Could you check a few things on this model? Use its own coordinates, in mm. Face numbers are marked on the shaded views. A direction names the side the tool comes from. Round coordinates to 2 decimals unless told otherwise and drop trailing zeros. Write each loop counter-clockwise with the first axis right and the second up, starting at its lowest first coordinate (ties: lowest second). Pieces come first, ordered by that corner, then holes. Notation, with made-up numbers: (58.25, 38.5) -> (83.25, 38.5) arc R14 ccw to (83.25, 63.5) -> close; hole circle Ø10 at (-11.75, 8). An arc over 180 degrees is marked (long way). Answer in a Markdown table with one row per item.
from build123d import *

# Parameters (mm, degrees)
SKETCH1_W           = 120
SKETCH1_H           = 37.194444444
BOSS_EXTRUDE4_DEPTH = 20
CUT_EXTRUDE15_DEPTH = 23
SKETCH10_W          = 11.898671916
SKETCH10_H          = 26.611218947
SKETCH10_W_2        = 10.049553983
SKETCH10_H_2        = 23.877740264
BOSS_EXTRUDE5_DEPTH = 30
SKETCH11_W          = 5.024776991
SKETCH11_H          = 23.877740264
BOSS_EXTRUDE6_DEPTH = 30
SKETCH12_W          = 4.765877192
SKETCH12_H          = 4.013370267
SKETCH12_H_2        = 4.515041551
CUT_EXTRUDE16_DEPTH = 16.868939526
FILLET2_R           = 5
SKETCH16_W          = 46.35727902
SKETCH16_H          = 19.765742142
CUT_EXTRUDE17_DEPTH = 5
FILLET3_R           = 5


with BuildPart() as part:
    # Sketch1 → Boss-Extrude4 (new body)
    with BuildSketch(Plane.XY):
        Polygon((36.833333333, 25.458333333), (36.833333333, 18.597222222), (60, 18.597222222), (60, -18.597222222), (68.25, -18.597222222), (72.583333333, 25.458333333), align=None)
        Rectangle(SKETCH1_W, SKETCH1_H)
    extrude(amount=BOSS_EXTRUDE4_DEPTH)

    # Sketch6 → Cut-Extrude15 (cut)
    with BuildSketch(Plane.XY.offset(20)):
        Polygon((51.910176302, 18.597222222), (36.833333333, 18.597222222), (36.833333333, 25.458333333), (72.583333333, 25.458333333), (68.25, -18.597222222), (55.010463364, -18.597222222), (60.177305366, 10.330093158), align=None)
    extrude(amount=-CUT_EXTRUDE15_DEPTH, mode=Mode.SUBTRACT)

    # Sketch10 → Boss-Extrude5 (add)
    with BuildSketch(Plane.ZY.offset(60)):
        with Locations((10.080396432, 0.080396432)):
            Rectangle(SKETCH10_W, SKETCH10_H)
        with Locations((10.120594648, 0.080396432)):
            Rectangle(SKETCH10_W_2, SKETCH10_H_2, mode=Mode.SUBTRACT)
    extrude(amount=BOSS_EXTRUDE5_DEPTH)

    # Sketch11 → Boss-Extrude6 (add)
    with BuildSketch(Plane.ZY.offset(60)):
        with Locations((12.632983144, 0.080396432)):
            Rectangle(SKETCH11_W, SKETCH11_H)
    extrude(amount=BOSS_EXTRUDE6_DEPTH)

    # Sketch12 → Cut-Extrude16 (cut, through all)
    with BuildSketch(Plane(origin=(0, 0, 4.131060474), x_dir=(-1, 0, 0), z_dir=(0, 0, -1))):
        with Locations((74.233976577, 5.142130655)):
            Rectangle(SKETCH12_W, SKETCH12_H)
        with Locations((74.233976577, -5.392966297)):
            Rectangle(SKETCH12_W, SKETCH12_H_2)
    extrude(amount=-CUT_EXTRUDE16_DEPTH, mode=Mode.SUBTRACT)

    # Fillet2
    fillet2_edges = [part.edges().sort_by_distance(p)[0] for p in [
        (-2.494768318, -18.597222222, 0),
        (56.043740834, 14.46365769, 0),
        (57.593884365, -4.133564532, 0),
        (-4.044911849, 18.597222222, 20),
        (-2.494768318, -18.597222222, 20),
        (55.010463364, -18.597222222, 10),
        (60.177305366, 10.330093158, 10),
        (51.910176302, 18.597222222, 10),
        (56.043740834, 14.46365769, 20),
        (57.593884365, -4.133564532, 20),
        (-4.044911849, 18.597222222, 0),
    ]]
    fillet(fillet2_edges, radius=FILLET2_R)

    # Sketch16 → Cut-Extrude17 (cut)
    with BuildSketch(Plane(origin=(0, 0, 0), x_dir=(-1, 0, 0), z_dir=(0, 0, -1))):
        Rectangle(SKETCH16_W, SKETCH16_H)
    extrude(amount=-CUT_EXTRUDE17_DEPTH, mode=Mode.SUBTRACT)

    # Fillet3
    fillet3_edges = [part.edges().sort_by_distance(p)[0] for p in [
        (23.17863951, -9.882871071, 2.5),
        (23.17863951, 9.882871071, 2.5),
        (-23.17863951, 9.882871071, 2.5),
        (-23.17863951, -9.882871071, 2.5),
    ]]
    fillet(fillet3_edges, radius=FILLET3_R)


solid = part.part
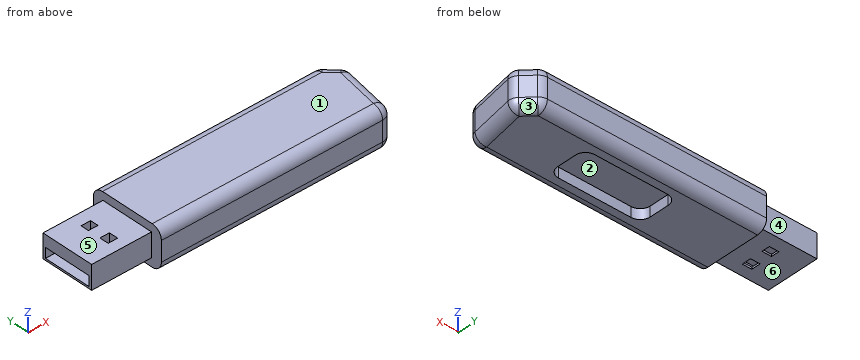
1) Imagine slicing it at B-B, the plane z = 6.75. Please give me the cut outline in (x, y), plus the area to 3 significant figures.
Findings:
| item | result |
|---|---|
| outline | (-90, -13.23) -> (-60, -13.23) -> (-60, -18.6) -> (50.82, -18.6) arc R5 ccw to (55.75, -14.48) -> (59.72, 7.76) arc R5 ccw to (58.33, 12.18) -> (53.37, 17.13) arc R5 ccw to (49.84, 18.6) -> (-60, 18.6) -> (-60, 13.39) -> (-90, 13.39) -> (-90, 12.02) -> (-60, 12.02) -> (-60, -11.86) -> (-90, -11.86) -> close |
| area | 4,440 mm^2 |
2) Please list where these lines run through material, in increasing order: line 1 (Z direction, x = 23, y = -1.5); line 2 (Z direction, x = 4, y = 14); line 3 (X direction, y = -7, z = 15.5).
Findings:
| item | result |
|---|---|
| line 1 | z = 5 to 20 |
| line 2 | z = 0.02 to 19.98 |
| line 3 | x = -90 to -76.62, -71.85 to 57.06 |
3) Thinking about a two-plate mould opening in X: for the marked faces 1, 2 and 3, which applies, +X half, -X half, draft (parallel to the pull), parting line (faces both ways), or undercut?
Findings:
| item | result |
|---|---|
| face 1 | draft |
| face 2 | undercut |
| face 3 | +X half |
4) For pin 1 (3.5 mm diameter, centred on y = -5, z = 12, fed in from +X); pin 2 (1.1 mm diameter, centred on y = -6, z = 5, fed in from +X); pin 3 (10 mm diameter, centred on y = -5, z = 12, fed in from +X), each with a flat end and sliding along its axis, tell me the tip position at first contact or that it passes through.
Findings:
| item | result |
|---|---|
| pin 1 | stops at x = 57.75 |
| pin 2 | stops at x = 57.36 |
| pin 3 | stops at x = 58.33 |
5) Imagine slicing it at D-D, the plane x = 6.5. Please give me the cut outline in (y, z), plus the area to 3 significant figures.
Findings:
| item | result |
|---|---|
| outline | (-18.6, 5) arc R5 ccw to (-13.6, 0) -> (-9.88, 0) -> (-9.88, 5) -> (9.88, 5) -> (9.88, 0) -> (13.6, 0) arc R5 ccw to (18.6, 5) -> (18.6, 15) arc R5 ccw to (13.6, 20) -> (-13.6, 20) arc R5 ccw to (-18.6, 15) -> close |
| area | 624 mm^2 |
6) Imagine slicing it at C-C, the plane x = 29. Please give me the cut outline in (y, z), plus the area to 3 significant figures.
Findings:
| item | result |
|---|---|
| outline | (-18.6, 5) arc R5 ccw to (-13.6, 0) -> (13.6, 0) arc R5 ccw to (18.6, 5) -> (18.6, 15) arc R5 ccw to (13.6, 20) -> (-13.6, 20) arc R5 ccw to (-18.6, 15) -> close |
| area | 722 mm^2 |
7) Imagine slicing it at A-A, the plane x = -80. Please give me the cut outline in (y, z).
Findings:
| item | result |
|---|---|
| outline | (-13.23, 4.13) -> (13.39, 4.13) -> (13.39, 16.03) -> (-13.23, 16.03) -> close; hole (-11.86, 5.1) -> (12.02, 5.1) -> (12.02, 10.12) -> (-11.86, 10.12) -> close |
8) For the marked faces 4, 5 and 6, which set-ups out of +Z, -Z, +X, -X, +Y, -Y let a thin tool reach every point of the face, with its end or its side?
Findings:
| item | result |
|---|---|
| face 4 | +Z, -Z, -X, +Y |
| face 5 | +Z, -X, +Y, -Y |
| face 6 | -Z, -X, +Y, -Y |
